CAD build for the part. Positions are in the model's coordinates, mm. A direction names the side the tool comes from. Give positions to 0.01 mm unless a question says otherwise; leave off trailing zeros. Loops run counter-clockwise (first coordinate to the right, second up) from the corner with the lowest first, then second, coordinate; pieces in that order, holes last. Notation, with made-up numbers: (-26.75, 12.5) -> (-14.75, 12.5) arc R17 ccw to (-14.75, 30.5) -> close; hole circle Ø7 at (76, 9.25). An arc over 180 degrees is marked (long way). Use one line per item in the form item = value.
```python
from build123d import *

# Parameters (mm, degrees)
SKETCH1_R           = 6.5
BOSS_EXTRUDE1_DEPTH = 4
BOSS_EXTRUDE2_DEPTH = 4
SKETCH3_R           = 2.1
CUT_EXTRUDE1_DEPTH  = 30.683160209
FILLET1_R           = 3


with BuildPart() as part:
    # Sketch1 → Boss-Extrude1 (new body)
    with BuildSketch(Plane.XY):
        Polygon((19.5, 3.8), (21.5, 3.8), (21.5, -3.8), (19.5, -3.8), (19.5, -15), (-19.5, -15), (-19.5, -3.8), (-21.5, -3.8), (-21.5, 3.8), (-19.5, 3.8), (-19.5, 15), (19.5, 15), align=None)
        Circle(SKETCH1_R, mode=Mode.SUBTRACT)
    extrude(amount=BOSS_EXTRUDE1_DEPTH)

    # Sketch2 → Boss-Extrude2 (add)
    with BuildSketch(Plane.XY.offset(4)):
        with BuildLine():
            Line((-21.5, 3.8), (-21.5, -3.8))
            ThreePointArc((-21.5, -3.8), (-25.3, 0), (-21.5, 3.8))
        make_face()
    boss_extrude2 = extrude(amount=-BOSS_EXTRUDE2_DEPTH)

    # Sketch3 → Cut-Extrude1 (cut, through all)
    with BuildSketch(Plane.XY.offset(4)):
        with Locations((-21.5, 0)):
            Circle(SKETCH3_R)
    cut_extrude1 = extrude(amount=-CUT_EXTRUDE1_DEPTH, mode=Mode.SUBTRACT)

    # Mirror1: Boss-Extrude2, Cut-Extrude1 across plane
    add(boss_extrude2.mirror(Plane.ZY))
    add(cut_extrude1.mirror(Plane.ZY), mode=Mode.SUBTRACT)

    # Fillet1
    fillet1_edges = [part.edges().sort_by_distance(p)[0] for p in [
        (19.5, -15, 2),
        (-19.5, -15, 2),
        (-19.5, 15, 2),
        (19.5, 15, 2),
    ]]
    fillet(fillet1_edges, radius=FILLET1_R)


solid = part.part
```
1. Mould opens along Y. For faces 1 (the flat face through (20, 3.8, 2)), 2 (the flat face through (0, -15, 2)), 3 (the cylindrical face through (-19.497, 0.631, 2.028)), 4 (the cylindrical face through (19.497, 0.631, 2.028)) say: pulls with the +Y half, pulls with the -Y half, needs draft (parallel to the pull), parting line crosses it, or undercut.
Result sheet:
face_1 = pulls with the +Y half
face_2 = pulls with the -Y half
face_3 = undercut
face_4 = undercut
2. Cut at C-C, the plane z = 1.6. Write the cut outline in (x, y).
Result sheet:
outline = (-21.5, -3.8) -> (-19.5, -3.8) -> (-19.5, -12) arc R3 ccw to (-16.5, -15) -> (16.5, -15) arc R3 ccw to (19.5, -12) -> (19.5, -3.8) -> (21.5, -3.8) arc R3.8 ccw to (21.5, 3.8) -> (19.5, 3.8) -> (19.5, 12) arc R3 ccw to (16.5, 15) -> (-16.5, 15) arc R3 ccw to (-19.5, 12) -> (-19.5, 3.8) -> (-21.5, 3.8) arc R3.8 ccw to start; hole circle Ø4.2 at (-21.5, 0); hole circle Ø13 at (0, 0); hole circle Ø4.2 at (21.5, 0)
3. Drill centre lines: line 1 (Y direction, x = 0, z = 2.8); line 2 (X direction, y = -1.75, z = 2.6); line 3 (X direction, y = -12.75, z = 0.95). Where is each one in solid material? Low to high.
Result sheet:
line_1 = -15 to -6.5, 6.5 to 15
line_2 = -24.87 to -22.66, -20.34 to -6.26, 6.26 to 20.34, 22.66 to 24.87
line_3 = -19.4 to 19.4
4. Cut at A-A, the plane y = 0. Write the cut outline in (x, z), then the cut area to 3 significant figures.
Result sheet:
outline = (-25.3, 0) -> (-23.6, 0) -> (-23.6, 4) -> (-25.3, 4) -> close; (-19.4, 0) -> (-6.5, 0) -> (-6.5, 4) -> (-19.4, 4) -> close; (6.5, 0) -> (19.4, 0) -> (19.4, 4) -> (6.5, 4) -> close; (23.6, 0) -> (25.3, 0) -> (25.3, 4) -> (23.6, 4) -> close
area = 117 mm^2
5. Drop flat-ended pins along their axis: P1, Ø1, axis at x = 20.5, z = 1, coming from the +Y side; P2, Ø2, axis at y = -6, z = 2, coming from the +X side; P3, Ø2, axis at y = 2, z = 3, coming from the -X side; P4, Ø2.5, axis at x = -21.5, y = 0, coming from the +Z side. Give the stop position or say it passes through.
Result sheet:
P1 = 3.8
P2 = 19.5
P3 = -25.17
P4 = through
6. Cut at D-D, the plane x = 5.5. Write the cut outline in (y, z).
Result sheet:
outline = (-15, 0) -> (-3.46, 0) -> (-3.46, 4) -> (-15, 4) -> close; (3.46, 0) -> (15, 0) -> (15, 4) -> (3.46, 4) -> close
7. Cut at B-B, the plane x = 0. Write the cut outline in (y, z).
Result sheet:
outline = (-15, 0) -> (-6.5, 0) -> (-6.5, 4) -> (-15, 4) -> close; (6.5, 0) -> (15, 0) -> (15, 4) -> (6.5, 4) -> close
8. Tool access for faces 5 (the flat face through (21, -3.8, 2)), 6 (the flat face through (-19.5, 8, 2)), 7 (the flat face through (-19.5, -8, 2)), 8 (the flat face through (-6, 4, 4)), 9 (the cylindrical face through (-5.158, -3.955, 1.972)): list every direction of +Z, -Z, +X, -X, +Y, -Y with a clear straight run to the whole face (end or side of a thin tool).
Result sheet:
face_5 = +Z, -Z, +X, -Y
face_6 = +Z, -Z, -X, +Y
face_7 = +Z, -Z, -X, -Y
face_8 = +Z, +X, -X, +Y, -Y
face_9 = +Z, -Z
